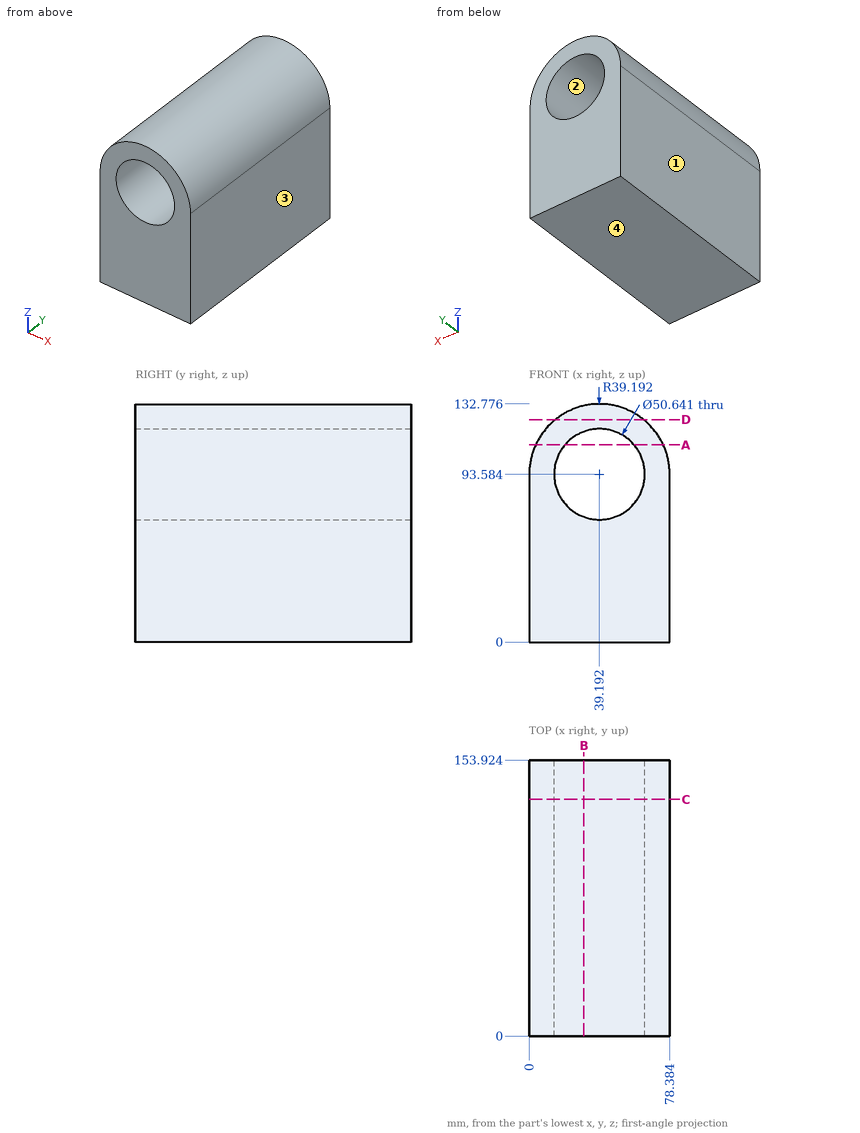
Geometry: see drawing. Coordinates: mm, zero at the bounding-box minimum. Coordinates: 2 decimals unless noted, no trailing zeros. Order: outer loops, then holes, each group sorted by start corner. A loop starts at its lowest first (then second) coordinate and runs counter-clockwise, first axis right, second up. Notation, with made-up numbers: (13.25, -15) -> (54.25, -15) arc R12 cw to (54.25, -1) -> close; hole circle Ø1 at (73, 28). An arc over 180 degrees is marked (long way). Write each question's results on one line, items separated by ' | '. Start each with the question number.
1) Cut plane C-C, the plane y = 132. Output: boundary loops of the cut face in (x, z).
2) Cut plane B-B, the plane x = 30.5. Output: boundary loops of the cut face in (y, z) (1 decimal).
3) Material intervals for line 1 along Z through (x, y) = (38, 117.5) (1 decimal); line 2 along X through (y, z) = (78.5, 71) (1 decimal); line 3 along X through (y, z) = (95.5, 102) (1 decimal), sorted ascending.
4) Cut plane A-A, the plane z = 110. Output: boundary loops of the cut face in (x, y) (1 decimal), and give its area (3 significant figures).
5) Cut plane D-D, the plane z = 124. Output: boundary loops of the cut face in (x, y), and give its area (3 significant figures).
6) First-contact query: pin 1 (8 mm diameter, centred on x = 56, y = 89.5, fed in from +Z). Flat tip, straight axial feed; report the tip coordinate or a pass-through.
7) Mould query, pull axis X, two halves, no side actions, for the marked faces 1, 2, 3 and 4. Classes: released by +X, released by -X, zero draft, split by the parting line, or undercut.
Checks:
1) outline: (0, 0) -> (78.38, 0) -> (78.38, 93.58) arc R39.19 ccw to (0, 93.58) -> close; hole circle Ø50.64 at (39.19, 93.58)
2) outline: (0, 0) -> (153.9, 0) -> (153.9, 69.8) -> (0, 69.8) -> close; (0, 117.4) -> (153.9, 117.4) -> (153.9, 131.8) -> (0, 131.8) -> close
3) line 1: 0 to 68.3, 118.9 to 132.8 | line 2: 0 to 27.7, 50.6 to 78.4 | line 3: 0.9 to 15.3, 63.1 to 77.5
4) outline: (3.6, 0) -> (19.9, 0) -> (19.9, 153.9) -> (3.6, 153.9) -> close; (58.5, 0) -> (74.8, 0) -> (74.8, 153.9) -> (58.5, 153.9) -> close | area: 5,020 mm^2
5) outline: (14.48, 0) -> (63.91, 0) -> (63.91, 153.92) -> (14.48, 153.92) -> close | area: 7,610 mm^2
6) pin 1: z = 130.62
7) face 1: released by -X | face 2: undercut | face 3: released by +X | face 4: zero draft
